Could you check a few things on this model? Use its own coordinates, in mm. Round coordinates to 2 decimals unless told otherwise and drop trailing zeros. Write each loop counter-clockwise with the first axis right and the second up, starting at its lowest first coordinate (ties: lowest second). Pieces come first, ordered by that corner, then holes. Notation, with made-up numbers: (83, 47.25) -> (125, 47.25) arc R30 cw to (125, 71.25) -> close; hole circle Ø9 at (21, 48.25). An arc over 180 degrees is marked (long way). One line per question, with ' | ' between items. Start each with the question number.
1. Imagine slicing it at C-C, the plane y = 4.5. List the corners of the cut face in (x, z) for me.
2. Imagine slicing it at A-A, the plane x = -2.5. List the corners of the cut face in (y, z) for me, and give its area (3 significant figures).
3. If I drill on line 1 along Z through (x, y) = (-2.5, 3.85); line 2 along Z through (x, y) = (-1.35, 1.5), over which ranges is the centre line in solid material (lowest first)? Write a range as [from, to].
4. Thinking about a two-plate mould opening in Z: for faces 1 (the flat face through (0, 2, 10)), 2 (the flat face through (-3, 3, 0)), 3 (the cylindrical face through (-1.69, 2.46, 0.95)), which applies, released by +Z, released by -Z, zero draft, split by the parting line, or undercut?
5. Imagine slicing it at B-B, the plane z = 2.5. List the corners of the cut face in (x, y) for me, and give its area (3 significant figures).
from build123d import *

# Parameters (mm, degrees)
SCHIZZO1_W                   = 5
SCHIZZO1_H                   = 5
ESTRUSIONE_ESTRUSIONE1_DEPTH = 20
SCHIZZO2_R                   = 1.75
TAGLIO_ESTRUSIONE1_DEPTH     = 22.213203436


with BuildPart() as part:
    # Schizzo1 → Estrusione-Estrusione1 (new body)
    with BuildSketch(Plane.XY):
        with Locations((-2.5, 2.5)):
            Rectangle(SCHIZZO1_W, SCHIZZO1_H)
    extrude(amount=ESTRUSIONE_ESTRUSIONE1_DEPTH)

    # Schizzo2 → Taglio-Estrusione1 (cut, through all)
    with BuildSketch(Plane(origin=(0, 0, 0), x_dir=(-1, 0, 0), z_dir=(0, -1, 0))):
        with Locations((2.5, -27.5)):
            Circle(SCHIZZO2_R)
        with Locations(Location((2.5, -2.5, 0), (0, 0, 180))):
            Circle(SCHIZZO2_R)
    extrude(amount=-TAGLIO_ESTRUSIONE1_DEPTH, mode=Mode.SUBTRACT)


solid = part.part
Geometry results:
1) outline: (-5, 0) -> (0, 0) -> (0, 20) -> (-5, 20) -> close; hole circle Ø3.5 at (-2.5, 2.5)
2) outline: (0, 0) -> (5, 0) -> (5, 0.75) -> (0, 0.75) -> close; (0, 4.25) -> (5, 4.25) -> (5, 20) -> (0, 20) -> close | area: 82.5 mm2
3) line 1: z = [0, 0.75], [4.25, 20] | line 2: z = [0, 1.18], [3.82, 20]
4) face 1: zero draft | face 2: released by -Z | face 3: undercut
5) outline: (-5, 0) -> (-4.25, 0) -> (-4.25, 5) -> (-5, 5) -> close; (-0.75, 0) -> (0, 0) -> (0, 5) -> (-0.75, 5) -> close | area: 7.50 mm2
